```python
from build123d import *

# Parameters (mm, degrees)
SKETCH5_R          = 0.889
CUT_EXTRUDE1_DEPTH = 12.7


with BuildPart() as part:
    # Sketch2 → Revolve1 (revolve)
    with BuildSketch(Plane.XY):
        Polygon((-38.1, -5.147815534), (-44.45, -5.147815534), (-44.45, 1.202184466), (-3.175, 1.202184466), (-3.175, -5.147815534), (-34.925, -5.147815534), align=None)
    revolve(axis=Axis((0, 49.967071373, 0), (0, -1, 0)))

    # Sketch5 → Cut-Extrude1 (cut)
    with BuildSketch(Plane(origin=(0, 1.202184466, 0), x_dir=(1, 0, 0), z_dir=(0, 1, 0))):
        with Locations((-41.275, 0)):
            Circle(SKETCH5_R)
        with Locations((-35.745198541, 20.6375)):
            Circle(SKETCH5_R)
        with Locations((-20.6375, 35.745198541)):
            Circle(SKETCH5_R)
        with Locations((0, 41.275)):
            Circle(SKETCH5_R)
        with Locations((20.6375, 35.745198541)):
            Circle(SKETCH5_R)
        with Locations((35.745198541, 20.6375)):
            Circle(SKETCH5_R)
        with Locations((41.275, 0)):
            Circle(SKETCH5_R)
        with Locations((35.745198541, -20.6375)):
            Circle(SKETCH5_R)
        with Locations((20.6375, -35.745198541)):
            Circle(SKETCH5_R)
        with Locations((0, -41.275)):
            Circle(SKETCH5_R)
        with Locations((-20.6375, -35.745198541)):
            Circle(SKETCH5_R)
        with Locations((-35.745198541, -20.6375)):
            Circle(SKETCH5_R)
    extrude(amount=-CUT_EXTRUDE1_DEPTH, mode=Mode.SUBTRACT)


solid = part.part
```
Check sheet for the modelled part. Datum: model origin and axes. Units: mm. Give positions to 0.01 mm unless a question says otherwise; leave off trailing zeros. Loops run counter-clockwise (first coordinate to the right, second up) from the corner with the lowest first, then second, coordinate; pieces in that order, holes last. Notation, with made-up numbers: M 2.25,-1 L 7.25,-1 A11 ccw 7.25,4 Z; hole C 50,31.25 d1. An arc over 180 degrees is marked long. Answer as CSV lines item,"result".
Item 1: Scan lines: L1, parallel to X at y = -1, z = 0 (3 decimals); L2, parallel to X at y = -2, z = 36; L3, parallel to X at y = -2.25, z = -35. Record each from-to range of solid material in increasing order.
Reply:
L1,"-44.45 to -42.164, -40.386 to -3.175, 3.175 to 40.386, 42.164 to 44.45"
L2,"-26.07 to -21.49, -19.79 to 19.79, 21.49 to 26.07"
L3,"-27.4 to -21.12, -20.15 to 20.15, 21.12 to 27.4"
Item 2: Sectioned sample at A-A, the plane y = -2.25. State how many separate pieces and enclosed holes the cut face has, then the cut area to 3 significant figures.
Reply:
separate pieces,"1"
enclosed holes,"13"
area,"6,150 mm^2"
Item 3: Draft check along Z on faces 1 (the face through (1, 1.202, 9)), 2 (the face through (-42.397, -1.928, -13.352)), 3 (the face through (0.69, -2.02, 3.1)). Enter one of: pulls with the +Z half, pulls with the -Z half, needs draft (parallel to the pull), parting line crosses it, or undercut.
Reply:
face 1,"needs draft"
face 2,"parting line crosses it"
face 3,"undercut"
Item 4: Sectioned sample at B-B, the plane x = 23.5. Enter the section's corners in (y, z).
Reply:
outline,"M -5.15,-37.73 L 1.2,-37.73 L 1.2,37.73 L -5.15,37.73 Z"
Item 5: Sectioned sample at C-C, the plane z = 38. Enter the section's corners in (x, y).
Reply:
outline,"M -23.06,-5.15 L 23.06,-5.15 L 23.06,1.2 L -23.06,1.2 Z"
Item 6: Depth check by flat-ended pin: pin 1 Ø2.5 at (x, z) = (-35.75, 20.64) entering from -Y; pin 2 Ø3 at (y, z) = (-3, 20.5) entering from -X; pin 3 Ø3 at (y, z) = (-1, 18.5) entering from +X. Enter the tip coordinate at first touch or a pass-through.
Reply:
pin 1,"y = -5.15"
pin 2,"x = -40.18"
pin 3,"x = 41.07"
